Build history of the part. All positions in model axes, mm. Give positions to 0.01 mm unless a question says otherwise; leave off trailing zeros. Order: outer loops, then holes, each group sorted by start corner. A loop starts at its lowest first (then second) coordinate and runs counter-clockwise, first axis right, second up. Notation, with made-up numbers: (4, 1.5) - (8, 1.5) arc R25 cw to (8, 18.5) - close; hole circle Ø3 at (24.25, 86). An arc over 180 degrees is marked (long way). One line per item, written item: value.
```python
from build123d import *

# Parameters (mm, degrees)
F0_R      = 47.5
F1_DEPTH  = 45
F2_W      = 40.64
F2_H      = 40.64
F3_DEPTH  = 35
F4_R      = 6
F6_DEPTH  = 10.001
F7_W      = 7.9080420285
F7_H      = 7.9080420285
F8_DEPTH  = 35
F9_R      = 4
F10_DEPTH = 10.001
F11_DEPTH = 35
F12_R     = 2.5
F13_DEPTH = 10.001


with BuildPart() as f1:
    # F0 (on Top) → F1 (new body)
    with BuildSketch(Plane.XY):
        Circle(F0_R)
    extrude(amount=F1_DEPTH)

    # F2 (on face) → F3 (cut)
    with BuildSketch(Plane.XY.offset(45)):
        Rectangle(F2_W, F2_H)
    extrude(amount=-F3_DEPTH, mode=Mode.SUBTRACT)

    # F4 (on face) → F6 (cut, through all)
    with BuildSketch(Plane.XY.offset(10)):
        Circle(F4_R)
    extrude(amount=-F6_DEPTH, mode=Mode.SUBTRACT)

    # F7 (on face) → F8 (cut)
    with BuildSketch(Plane.XY.offset(45)):
        Polygon((37.3080420285, 37.3080420285), (37.3080420285, 29.4), (29.4, 29.4), (29.4, -29.4), (37.3080420285, -29.4), (37.3080420285, -37.3080420285), (49.4, -37.3080420285), (49.4, 37.3080420285), align=None)
        with Locations((33.3540210142, 33.3540210142)):
            Rectangle(F7_W, F7_H)
        Polygon((-29.4, 29.4), (29.4, 29.4), (29.4, 37.3080420285), (37.3080420285, 37.3080420285), (37.3080420285, 49.4), (-37.3080420285, 49.4), (-37.3080420285, 37.3080420285), (-29.4, 37.3080420285), align=None)
        Polygon((-29.4, -29.4), (-29.4, 29.4), (-37.3080420285, 29.4), (-37.3080420285, 37.3080420285), (-49.4, 37.3080420285), (-49.4, -37.3080420285), (-37.3080420285, -37.3080420285), (-37.3080420285, -29.4), align=None)
        with Locations((-33.3540210142, 33.3540210142)):
            Rectangle(F7_W, F7_H)
        Polygon((29.4, -37.3080420285), (29.4, -29.4), (-29.4, -29.4), (-29.4, -37.3080420285), (-37.3080420285, -37.3080420285), (-37.3080420285, -49.4), (37.3080420285, -49.4), (37.3080420285, -37.3080420285), align=None)
        with Locations((33.3540210142, -33.3540210142)):
            Rectangle(F7_W, F7_H)
        with Locations((-33.3540210142, -33.3540210142)):
            Rectangle(F7_W, F7_H)
    extrude(amount=-F8_DEPTH, mode=Mode.SUBTRACT)

    # F9 (on face) → F10 (cut, through all)
    with BuildSketch(Plane.XY.offset(10)):
        with Locations((0, 39.35)):
            Circle(F9_R)
        with Locations((39.35, 0)):
            Circle(F9_R)
        with Locations((0, -39.35)):
            Circle(F9_R)
        with Locations((-39.35, 0)):
            Circle(F9_R)
    extrude(amount=-F10_DEPTH, mode=Mode.SUBTRACT)

    # F11 (cut): a face of the model
    f11_faces = [f1.faces().sort_by_distance(p)[0] for p in [
        (0, -28.5684424253, 45),
    ]]
    extrude(f11_faces, amount=-F11_DEPTH, mode=Mode.SUBTRACT)

    # F12 (on face) → F13 (cut, through all)
    with BuildSketch(Plane(origin=(0, 0, 0), x_dir=(1, 0, 0), z_dir=(0, 0, -1))):
        with Locations((0, 24.86)):
            Circle(F12_R)
        with Locations((24.86, 0)):
            Circle(F12_R)
        with Locations((0, -24.86)):
            Circle(F12_R)
        with Locations((-24.86, 0)):
            Circle(F12_R)
    extrude(amount=-F13_DEPTH, mode=Mode.SUBTRACT)


solid = f1.part
```
(1) Drill centre lines: line 1 (Y direction, x = 0, z = 6); line 2 (X direction, y = 3, z = 9); line 3 (Y direction, x = -1, z = 8). Where is each one in solid material? Low to high.
Completed:
line 1: -47.5 to -43.35, -35.35 to -27.36, -22.36 to -6, 6 to 22.36, 27.36 to 35.35, 43.35 to 47.5
line 2: -47.41 to -42, -36.7 to -5.2, 5.2 to 36.7, 42 to 47.41
line 3: -47.49 to -43.22, -35.48 to -27.15, -22.57 to -5.92, 5.92 to 22.57, 27.15 to 35.48, 43.22 to 47.49
(2) Pin check, flat tips, straight feed: P1, Ø5, axis at x = -39.35, y = 0, coming from the +Z side; P2, Ø3, axis at x = 11.5, z = 2.5, coming from the -Y side; P3, Ø5, axis at x = -21, z = 5.5, coming from the -Y side; P4, Ø6, axis at x = 1, z = 8, coming from the -Y side. Stop position of each tip, or through.
Completed:
P1: through
P2: y = -46.44
P3: y = -43.75
P4: y = -47.5
(3) Slice it at A-A, the plane x = 0. Give the cut face in (y, z).
Completed:
outline: (-47.5, 0) - (-43.35, 0) - (-43.35, 10) - (-47.5, 10) - close; (-35.35, 0) - (-27.36, 0) - (-27.36, 10) - (-35.35, 10) - close; (-22.36, 0) - (-6, 0) - (-6, 10) - (-22.36, 10) - close; (6, 0) - (22.36, 0) - (22.36, 10) - (6, 10) - close; (27.36, 0) - (35.35, 0) - (35.35, 10) - (27.36, 10) - close; (43.35, 0) - (47.5, 0) - (47.5, 10) - (43.35, 10) - close
(4) Slice it at D-D, the plane x = -39.35. Give the cut face in (y, z).
Completed:
outline: (-26.61, 0) - (-4, 0) - (-4, 10) - (-26.61, 10) - close; (4, 0) - (26.61, 0) - (26.61, 10) - (4, 10) - close
(5) Slice it at B-B, the plane z = 5. Count the separate pieces of the cut face and the enclosed holes in it, and give its area (3 significant figures).
Completed:
separate pieces: 1
enclosed holes: 9
area: 6,700 mm²
